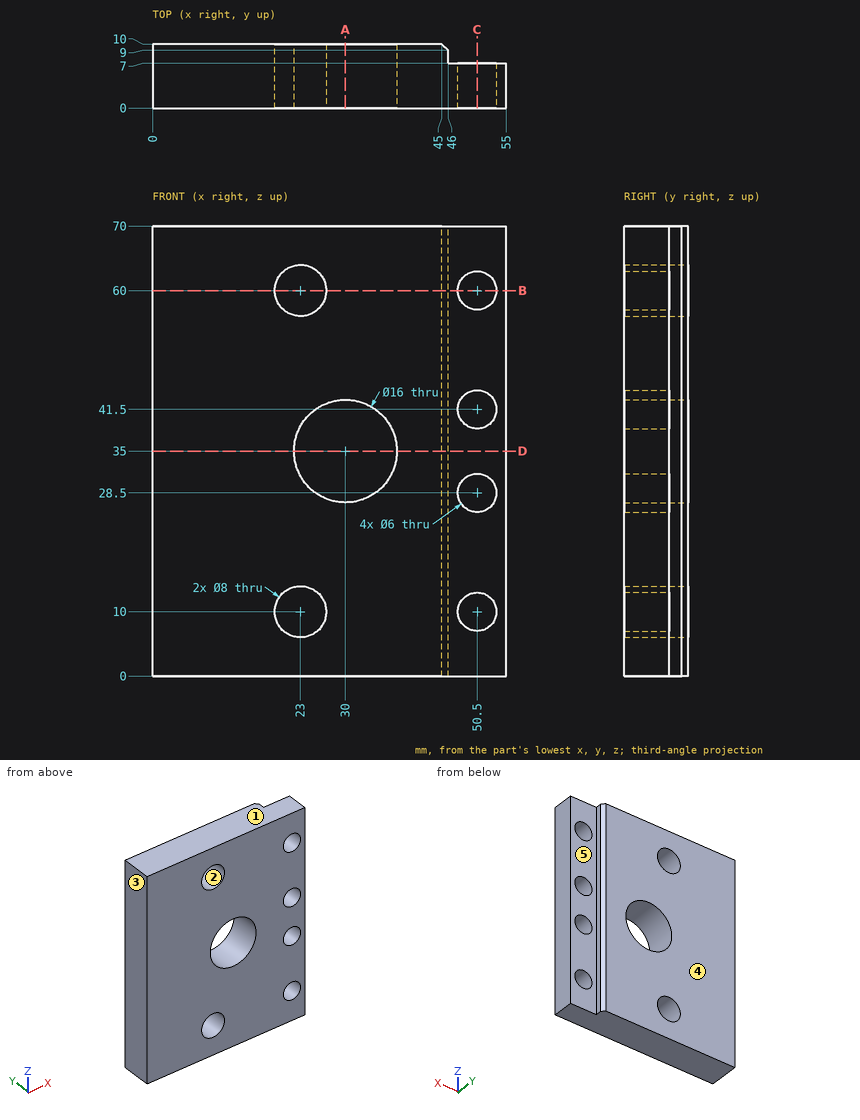
Design review of the part shown in the three views and the two pictorial views. Dimensions are in mm from the part's minimum x, y and z. A direction names the side the tool comes from. Round coordinates to 2 decimals unless told otherwise and drop trailing zeros. Write each loop counter-clockwise with the first axis right and the second up, starting at its lowest first coordinate (ties: lowest second). Pieces come first, ordered by that corner, then holes.
Item 1: Wall thickness on L1, parallel to X at y = 4.25, z = 60; L2, parallel to Z at x = 50.5, y = 3; L3, parallel to Z at x = 49.5, y = 1.5: over which ranges is each line inside the solid? List them lowest first.
Item 2: Consider section A-A on x = 30. Give the boundary of the cut face in (y, z).
Item 3: Consider section C-C on x = 50.5. Give the boundary of the cut face in (y, z).
Item 4: For pin 1 Ø2 at (x, z) = (45.5, 23) entering from -Y; pin 2 Ø2.5 at (x, z) = (49.5, 27.5) entering from +Y; pin 3 Ø0.6 at (y, z) = (8.5, 48) entering from +X, all flat-tipped, find the tip position at first contact; note any pin that passes through.
Item 5: Consider section B-B on z = 60. Give the boundary of the cut face in (x, y).
Item 6: Draft analysis for pull direction Z (two halves, no side actions). For the marked faces 1, 2 and 3, state which applies: released by +Z, released by -Z, zero draft, split by the parting line, or undercut.
Item 7: For the marked faces 4 and 5, list the 3-axis set-ups (+Z, -Z, +X, -X, +Y, -Y) from which the entire face can be reached by the end or side of a thin tool; tool diameter is ignored.
Item 8: Consider section D-D on z = 35. Give the boundary of the cut face in (x, y), and give its area (4 significant figures).
Check values:
1. L1: x = 0 to 19, 27 to 47.5, 53.5 to 55
1. L2: z = 0 to 7, 13 to 25.5, 31.5 to 38.5, 44.5 to 57, 63 to 70
1. L3: z = 0 to 7.17, 12.83 to 25.67, 31.33 to 38.67, 44.33 to 57.17, 62.83 to 70
2. outline: (0, 0) - (10, 0) - (10, 27) - (0, 27) - close; (0, 43) - (10, 43) - (10, 70) - (0, 70) - close
3. outline: (0, 0) - (7, 0) - (7, 7) - (0, 7) - close; (0, 13) - (7, 13) - (7, 25.5) - (0, 25.5) - close; (0, 31.5) - (7, 31.5) - (7, 38.5) - (0, 38.5) - close; (0, 44.5) - (7, 44.5) - (7, 57) - (0, 57) - close; (0, 63) - (7, 63) - (7, 70) - (0, 70) - close
4. pin 1: stops at y = 0
4. pin 2: passes through
4. pin 3: stops at x = 46
5. outline: (0, 0) - (19, 0) - (19, 10) - (0, 10) - close; (27, 0) - (47.5, 0) - (47.5, 7) - (46, 7) - (46, 9) - (45, 10) - (27, 10) - close; (53.5, 0) - (55, 0) - (55, 7) - (53.5, 7) - close
6. face 1: released by +Z
6. face 2: undercut
6. face 3: zero draft
7. face 4: +Z, -Z, +X, -X, +Y
7. face 5: +Z, -Z, +X, +Y
8. outline: (0, 0) - (22, 0) - (22, 10) - (0, 10) - close; (38, 0) - (55, 0) - (55, 7) - (46, 7) - (46, 9) - (45, 10) - (38, 10) - close
8. area: 362.5 mm2
